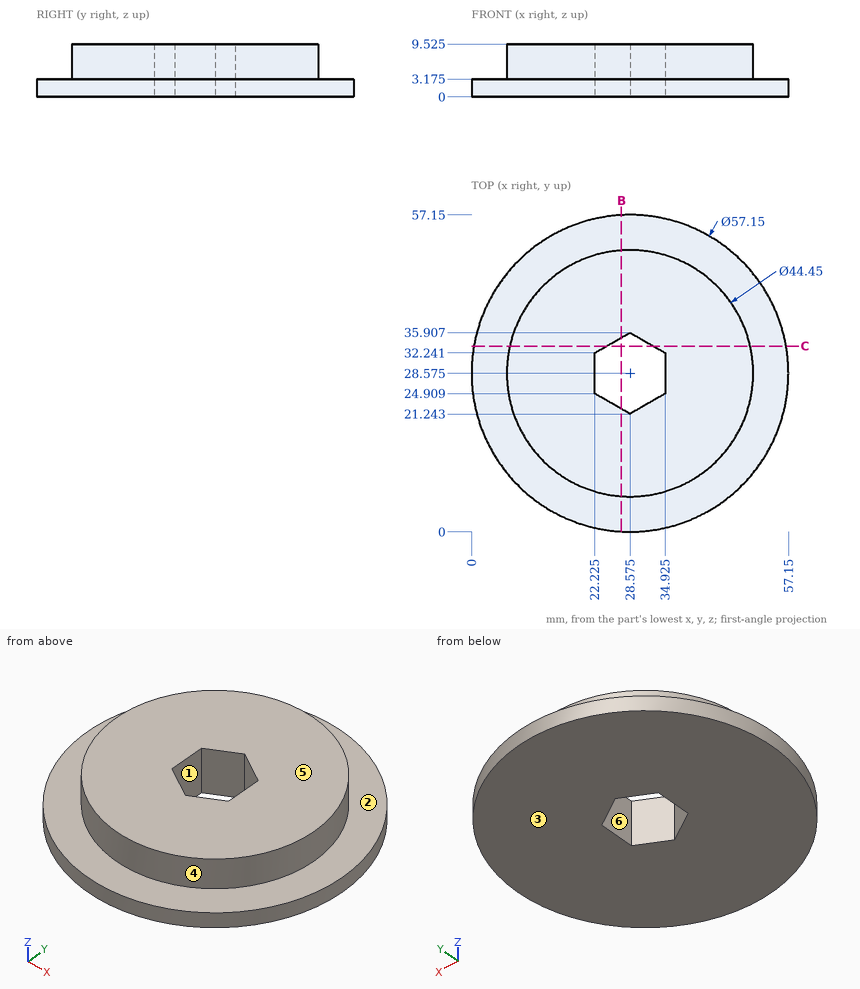
The figure shows three views and two pictorial views of one solid part (mm, origin at its lowest corner). Answer the questions. A direction names the side the tool comes from. Round coordinates to 2 decimals unless told otherwise and drop trailing zeros. Write each loop counter-clockwise with the first axis right and the second up, starting at its lowest first coordinate (ties: lowest second). Pieces come first, ordered by that corner, then holes. Notation, with made-up numbers: (76.25, 20) - (123.25, 20) arc R22 cw to (123.25, 41) - close; hole circle Ø10 at (24, 13.5). An arc over 180 degrees is marked (long way). Use one line per item in the form item = value. Start each with the question number.
Item 1: Determine the mould class of the marked faces 4, 5 and 6 for opening direction Y: +Y half, -Y half, draft (parallel to the pull), parting line (faces both ways), or undercut.
Item 2: A cutting plane is placed at C-C (y = 33.5). Write down the section's boundary in (x, z) (1 decimal).
Item 3: A cutting plane is placed at B-B (x = 27). Write down the section's boundary in (y, z) (1 decimal), plus the area to 3 significant figures.
Item 4: Flat-ended cylindrical pins translate along their axes: pin 1 Ø2 at (y, z) = (27, 4) entering from +X; pin 2 Ø2 at (y, z) = (19, 2.5) entering from -X; pin 3 Ø10 at (x, y) = (15, 51) entering from -Z; pin 4 Ø5 at (x, z) = (19, 3) entering from +Y. Find the tip coordinate at first contact, or state that the pin passes through.
Item 5: Find the intervals of material crossed by line 1 (X direction, y = 32.5, z = 3) (1 decimal); line 2 (Z direction, x = 11, y = 49.5) (1 decimal); line 3 (Y direction, x = 28, z = 2.25) (1 decimal), in increasing order. Write a range as [from, to].
Item 6: A tool of negligible diameter and unlimited length cuts with its end or side. For the marked faces 1, 2 and 3, from which of +Z, -Z, +X, -X, +Y, -Y can it reach the whole face along a straight path? Write none if from no direction.
The answers:
q1.face_4 = parting line
q1.face_5 = draft
q1.face_6 = undercut
q2.outline = (0.4, 0) - (24.4, 0) - (24.4, 9.5) - (6.9, 9.5) - (6.9, 3.2) - (0.4, 3.2) - close; (32.7, 0) - (56.7, 0) - (56.7, 3.2) - (50.2, 3.2) - (50.2, 9.5) - (32.7, 9.5) - close
q3.outline = (0, 0) - (22.2, 0) - (22.2, 9.5) - (6.4, 9.5) - (6.4, 3.2) - (0, 3.2) - close; (35, 0) - (57.1, 0) - (57.1, 3.2) - (50.7, 3.2) - (50.7, 9.5) - (35, 9.5) - close
q3.area = 340 mm^2
q4.pin_1 = 57.13
q4.pin_2 = 1.32
q4.pin_3 = 0
q4.pin_4 = 56.26
q5.line_1 = [0.3, 22.7], [34.5, 56.9]
q5.line_2 = [0, 3.2]
q5.line_3 = [0, 21.6], [35.6, 57.1]
q6.face_1 = +Z, -Z
q6.face_2 = +Z
q6.face_3 = -Z, +X, -X, +Y, -Y
